Can you work these out from the model? Positions are in its coordinate system, mm. A direction names the side the tool comes from. Give positions to 0.01 mm unless a question says otherwise; leave off trailing zeros. Write each loop counter-clockwise with the first axis right and the second up, starting at its lowest first coordinate (ties: lowest second). Pieces come first, ordered by that corner, then holes.
1. Thinking about a two-plate mould opening in Y: for faces 1 (the flat face through (0, 23.5, 1)), 2 (the flat face through (3, -25, 0)), 3 (the cylindrical face through (-42.47, -0.4, 1.49)), which applies, pulls with the +Y half, pulls with the -Y half, needs draft (parallel to the pull), parting line crosses it, or undercut?
2. If I drill on probe 1 along Y at (x, z) = (26, 1.85); probe 2 along X at (y, z) = (11, 1.9); probe 3 along X at (y, z) = (7, 1.4), over which ranges is the centre line in solid material (lowest first)?
3. On a 3-axis mill with a long thin cutter (end or side, diameter ignored), from which of +Z, -Z, +X, -X, +Y, -Y can I reach the whole of each face in a straight line? I mean faces 4 (the cylindrical face through (42.47, 0.4, 1.49)), 5 (the flat face through (32, 0, 1)). Say none if no direction works.
4. I'm going to push flat-ended pins straight in: pin 1 (0.6 mm diameter, centred on x = 4.5, z = 1, fed in from -Y); pin 2 (0.6 mm diameter, centred on y = 6.5, z = 1, fed in from -X); pin 3 (1.1 mm diameter, centred on x = 0, y = -30, fed in from -Z). Where does each tip first touch, or does it pass through?
5. Suppose I cut it at A-A (z = 1.65). Please give me the cut outline in (x, y) (3 decimals), and give its area (3 significant figures).
```python
from build123d import *

# Parameters (mm, degrees)
SKETCH1_W           = 64
SKETCH1_H           = 47
BOSS_EXTRUDE1_DEPTH = 2
FILLET1_R           = 1
SKETCH2_R           = 0.875
CUT_EXTRUDE1_DEPTH  = 55.981008251


with BuildPart() as part:
    # Sketch1 → Boss-Extrude1 (new body)
    # profile 1 of 2: a face of its own
    with BuildSketch(Plane.XY):
        with BuildLine():
            ThreePointArc((37, 27.5), (42.470090103, 0), (37, -27.5))
            ThreePointArc((37, -27.5), (0, -34.859757593), (-37, -27.5))
            ThreePointArc((-37, -27.5), (-42.470090103, 0), (-37, 27.5))
            ThreePointArc((-37, 27.5), (0, 34.859757593), (37, 27.5))
        make_face()
        with BuildLine():
            ThreePointArc((36, -25.5), (40.468092327, 0), (36, 25.5))
            ThreePointArc((36, 25.5), (0, 32.351769079), (-36, 25.5))
            ThreePointArc((-36, 25.5), (-40.468092327, 0), (-36, -25.5))
            ThreePointArc((-36, -25.5), (0, -32.351769079), (36, -25.5))
        make_face(mode=Mode.SUBTRACT)
    # profile 2 of 2: a face of its own
    with BuildSketch(Plane.XY):
        with BuildLine():
            ThreePointArc((36, -25.5), (0, -32.351769079), (-36, -25.5))
            ThreePointArc((-36, -25.5), (-40.468092327, 0), (-36, 25.5))
            ThreePointArc((-36, 25.5), (0, 32.351769079), (36, 25.5))
            ThreePointArc((36, 25.5), (40.468092327, 0), (36, -25.5))
        make_face()
        Rectangle(SKETCH1_W, SKETCH1_H, mode=Mode.SUBTRACT)
    extrude(amount=BOSS_EXTRUDE1_DEPTH)

    # Fillet1
    fillet1_edges = [part.edges().sort_by_distance(p)[0] for p in [
        (-42.470090103, 0, 0),
        (0, -34.859757593, 0),
        (0, 34.859757593, 0),
        (42.470090103, 0, 0),
    ]]
    fillet(fillet1_edges, radius=FILLET1_R)

    # Sketch2 → Cut-Extrude1 (cut, through all)
    with BuildSketch(Plane(origin=(0, 0, 0), x_dir=(-1, 0, 0), z_dir=(0, 0, -1))):
        with Locations((-38.75, 0)):
            Circle(SKETCH2_R)
        with Locations((0, -30)):
            Circle(SKETCH2_R)
        with Locations((38.75, 0)):
            Circle(SKETCH2_R)
    extrude(amount=-CUT_EXTRUDE1_DEPTH, mode=Mode.SUBTRACT)


solid = part.part
```
Checks:
1. face 1: undercut
1. face 2: needs draft
1. face 3: parting line crosses it
2. probe 1: y = -31.3 to -23.5, 23.5 to 31.3
2. probe 2: x = -41.62 to -32, 32 to 41.62
2. probe 3: x = -42.13 to -32, 32 to 42.13
3. face 4: +Z, -Z, +X
3. face 5: +Z, -Z
4. pin 1: stops at y = -34.77
4. pin 2: stops at x = -42.2
4. pin 3: passes through
5. outline: (-37, -27.5) arc R96.686 ccw to (37, -27.5) arc R71.861 ccw to (37, 27.5) arc R96.686 ccw to (-37, 27.5) arc R71.861 ccw to start; hole circle Ø1.75 at (-38.75, 0); hole (-32, -23.5) - (32, -23.5) - (32, 23.5) - (-32, 23.5) - close; hole circle Ø1.75 at (0, -30); hole circle Ø1.75 at (38.75, 0)
5. area: 2,190 mm2
